Autodesk Inventor part; units mm, degrees
ref_plane "YZ Plane" through (0, 0, 0) normal (1, 0, 0) x (0, 1, 0)
ref_plane "XZ Plane" through (0, 0, 0) normal (0, 1, 0) x (-1, 0, 0)
ref_plane "XY Plane" through (0, 0, 0) normal (0, 0, 1) x (1, 0, 0)
sketch "スケッチ1" plane through (0, 0, 0) normal (1, 0, 0) x (0, 1, 0)
  line L0 (-2.4757, 20.6884) -> (-6.5003, 29.5193)
  arc A0 (-6.5003, 29.5193) -> (5.7094, 31.948) centre (4.8303, 4.4621) ccw
  line L1 (5.7094, 31.948) -> (5.3706, 22.2491)
  line L2 (5.3706, 22.2491) -> (-2.4757, 20.6884)
  circle A1 centre (4.8303, -4.5379) radius 1.6
  circle A2 centre (4.8303, 13.4621) radius 1.6
  circle A3 centre (4.8303, 4.4621) radius 5.1
  point P0 (0, 0)
extrude "押し出し1" add sketch "スケッチ1" against normal blind 2.5
properties part number "belt_liner_v3_3DP_P-2-F" material "ABS プラスチック"
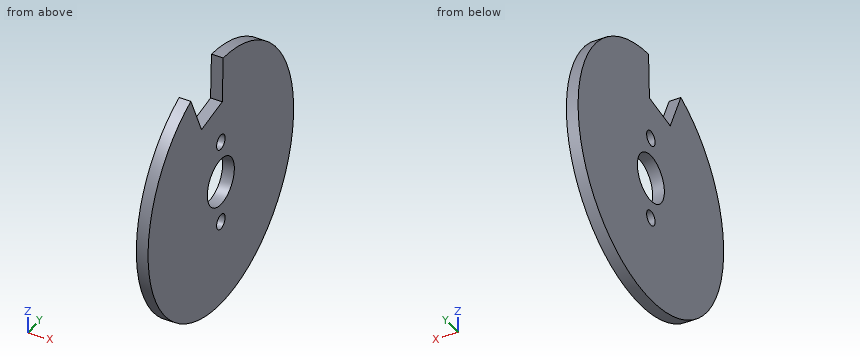
Verification items for the finished model (mm, model axes). Round coordinates to 2 decimals unless told otherwise and drop trailing zeros. Loops run counter-clockwise (first coordinate to the right, second up) from the corner with the lowest first, then second, coordinate; pieces in that order, holes last. Notation, with made-up numbers: (46, 87) -> (68, 87) arc R23 ccw to (68, 120) -> close; hole circle Ø11 at (-8, 24). An arc over 180 degrees is marked (long way). Answer as a JSON object with one key per item and string values.
Q1. Section check B-B (x = -0.7). Record the boundary of the cut face in (y, z).
Data:
{"outline": "(-6.5, 29.52) arc R27.5 ccw (long way) to (5.71, 31.95) -> (5.37, 22.25) -> (-2.48, 20.69) -> close; hole circle Ø10.2 at (4.83, 4.46); hole circle Ø3.2 at (4.83, -4.54); hole circle Ø3.2 at (4.83, 13.46)"}
Q2. Go/stop test with a flat-tipped pin: P1, Ø1.5, axis at x = -2, y = 6, coming from the -Z side. Record where the tip stops, or that it passes through.
Data:
{"P1": "stops at z = -23.03"}
Q3. Section check D-D (z = 26.5). Record the boundary of the cut face in (x, y), then the cut area to 3 significant figures.
Data:
{"outline": "(-2.5, -11.62) -> (0, -11.62) -> (0, -5.12) -> (-2.5, -5.12) -> close; (-2.5, 5.52) -> (0, 5.52) -> (0, 21.28) -> (-2.5, 21.28) -> close", "area": "55.6 mm2"}
Q4. Section check A-A (z = 2). Record the boundary of the cut face in (x, y), then the cut area to 3 significant figures.
Data:
{"outline": "(-2.5, -22.56) -> (0, -22.56) -> (0, 0.36) -> (-2.5, 0.36) -> close; (-2.5, 9.3) -> (0, 9.3) -> (0, 32.22) -> (-2.5, 32.22) -> close", "area": "115 mm2"}
Q5. Section check C-C (y = 20). Record the boundary of the cut face in (x, z).
Data:
{"outline": "(-2.5, -18.48) -> (0, -18.48) -> (0, 27.4) -> (-2.5, 27.4) -> close"}
Q6. Scan lines: line 1 (Y direction, x = -0.45, z = 4.5); line 2 (Y direction, x = -2.3, z = 2); line 3 (Y direction, x = -0.4, z = -6.5). Record each from-to range of solid material in increasing order. Write a range as from..to.
Data:
{"line 1": "y = -22.67..-0.27, 9.93..32.33", "line 2": "y = -22.56..0.36, 9.3..32.22", "line 3": "y = -20.39..30.05"}
